Part model, mm, in its own coordinate system. Face numbers are marked on the shaded views. Give positions to 0.01 mm unless a question says otherwise; leave off trailing zeros. Write each loop counter-clockwise with the first axis right and the second up, starting at its lowest first coordinate (ties: lowest second). Pieces come first, ordered by that corner, then holes. Notation, with made-up numbers: (24.5, 83.25) - (39.5, 83.25) arc R12 ccw to (39.5, 91.25) - close; hole circle Ø6 at (61, 81.25). An arc over 180 degrees is marked (long way). Answer as a JSON object with one key per item and string values. Group by question number.
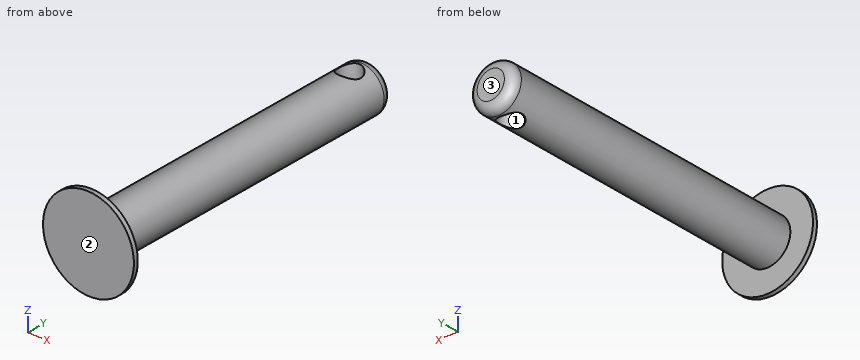
```python
from build123d import *

# Parameters (mm, degrees)
SCHIZZO1_R                    = 5
ESTRUSIONE_ESTRUSIONE1_DEPTH  = 70
RACCORDO1_R                   = 2
SCHIZZO2_R                    = 2.5
TAGLIO_ESTRUSIONE1_DEPTH      = 6
TAGLIO_ESTRUSIONE1_DEPTH_BACK = 6
SCHIZZO3_R                    = 10
ESTRUSIONE_ESTRUSIONE2_DEPTH  = 1


with BuildPart() as part:
    # Schizzo1 → Estrusione-Estrusione1 (new body)
    with BuildSketch(Plane(origin=(0, 0, 0), x_dir=(1, 0, 0), z_dir=(0, 1, 0))):
        Circle(SCHIZZO1_R)
    extrude(amount=ESTRUSIONE_ESTRUSIONE1_DEPTH)

    # Raccordo1
    raccordo1_edges = [part.edges().sort_by_distance(p)[0] for p in [
        (-5, 70, 0),
    ]]
    fillet(raccordo1_edges, radius=RACCORDO1_R)

    # Schizzo2 → Taglio-Estrusione1 (cut, two sides)
    with BuildSketch(Plane.XY) as taglio_estrusione1_sk:
        with Locations((0, 65)):
            Circle(SCHIZZO2_R)
    extrude(amount=TAGLIO_ESTRUSIONE1_DEPTH, mode=Mode.SUBTRACT)
    extrude(taglio_estrusione1_sk.sketch, amount=-TAGLIO_ESTRUSIONE1_DEPTH_BACK, mode=Mode.SUBTRACT)

    # Schizzo3 → Estrusione-Estrusione2 (add)
    with BuildSketch(Plane(origin=(0, 0, 0), x_dir=(-1, 0, 0), z_dir=(0, -1, 0))):
        Circle(SCHIZZO3_R)
    extrude(amount=ESTRUSIONE_ESTRUSIONE2_DEPTH)


solid = part.part
```
1) Saw through at D-D (x = -6). List the corners of the cut face in (y, z).
2) Drop flat-ended pins along their axis: P1, Ø5, axis at x = -0.5, y = 22.5, coming from the +Z side; P2, Ø8, axis at y = 6.5, z = 4, coming from the +X side; P3, Ø1, axis at x = -6.5, z = -4, coming from the +Y side. Give the stop position or say it passes through.
3) Drill centre lines: line 1 along X through (y, z) = (65, 0); line 2 along Y through (x, z) = (4.75, 4); line 3 along Y through (x, z) = (0, 1.5). Where is each one in solid material? Low to high. Write a range as from..to.
4) Saw through at A-A (x = 0). List the corners of the cut face in (y, z), and give its area (3 significant figures).
5) Two-plate mould, pull along Y, no slides. Class the marked faces 1, 2 and 3: +Y half, -Y half, draft (parallel to the pull), parting line (faces both ways), or undercut.
6) Saw through at B-B (z = 0). List the corners of the cut face in (x, y).
7) Saw through at C-C (y = 65). List the corners of the cut face in (x, z).
Checks:
{
 "1": {"outline": "(-1, -8) - (0, -8) - (0, 8) - (-1, 8) - close"},
 "2": {"P1": "z = 5", "P2": "x = 5", "P3": "y = 0"},
 "3": {"line 1": "-5..-2.5, 2.5..5", "line 2": "-1..0", "line 3": "-1..62.5, 67.5..70"},
 "4": {"outline": "(-1, -10) - (0, -10) - (0, -5) - (62.5, -5) - (62.5, 5) - (0, 5) - (0, 10) - (-1, 10) - close; (67.5, -5) - (68, -5) arc R2 ccw to (70, -3) - (70, 3) arc R2 ccw to (68, 5) - (67.5, 5) - close", "area": "668 mm2"},
 "5": {"face 1": "undercut", "face 2": "-Y half", "face 3": "+Y half"},
 "6": {"outline": "(-10, -1) - (10, -1) - (10, 0) - (5, 0) - (5, 68) arc R2 ccw to (3, 70) - (-3, 70) arc R2 ccw to (-5, 68) - (-5, 0) - (-10, 0) - close; hole circle Ø5 at (0, 65)"},
 "7": {"outline": "(-2.5, -4.33) - (-2.5, 4.33) arc R5 ccw to start; (2.5, -4.33) arc R5 ccw to (2.5, 4.33) - close"}
}
